Source: three-view drawing plus pictorial views. Frame: mm from the lowest corner of the part. Give positions to 0.01 mm unless a question says otherwise; leave off trailing zeros. Order: outer loops, then holes, each group sorted by start corner. A loop starts at its lowest first (then second) coordinate and runs counter-clockwise, first axis right, second up. Notation, with made-up numbers: M 78.25,64 L 127.25,64 A9 ccw 127.25,76 Z; hole C 61,31.25 d2. An arc over 180 degrees is marked long. Use CSV: the item, a comma, the result in double quotes.
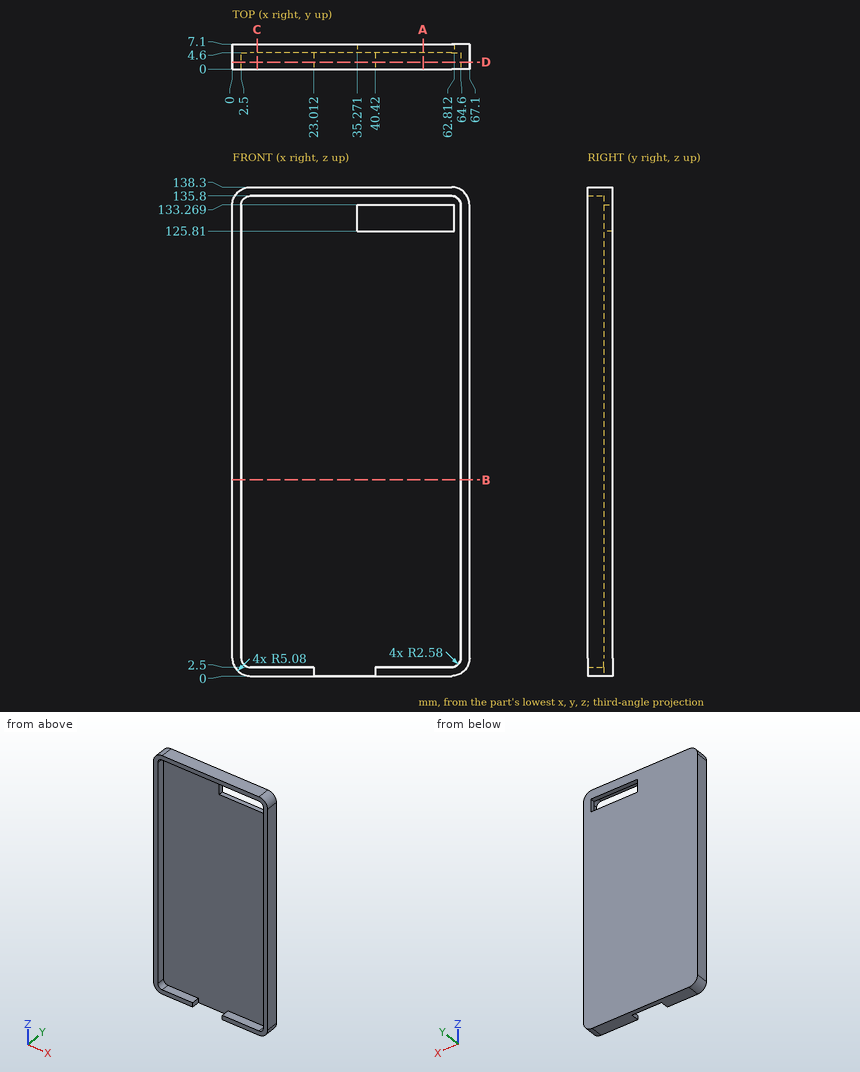
1. Section C-C, the plane x = 7. Return the cut outline in (y, z).
Answer:
outline,"M 0,0 L 7.1,0 L 7.1,138.3 L 0,138.3 L 0,135.8 L 4.6,135.8 L 4.6,2.5 L 0,2.5 Z"
2. Line query: line 1 (Z direction, x = 54.5, y = 6); line 2 (X direction, y = 4, z = 72); line 3 (Z direction, x = 57, y = 0.5). Output: solid intervals per line, ascending.
Answer:
line 1,"0 to 125.81, 133.27 to 138.3"
line 2,"0 to 2.5, 64.6 to 67.1"
line 3,"0 to 2.5, 135.8 to 138.3"
3. Pin query (flat end, axial travel): pin 1 Ø3 at (y, z) = (5.5, 129.5) entering from -X; pin 2 Ø18.5 at (x, z) = (32.5, 92.5) entering from -Y; pin 3 Ø1.2 at (y, z) = (2, 1) entering from -X; pin 4 Ø0.8 at (y, z) = (1.5, 1) entering from +X. Return the tip coordinate at first contact, or that it passes through.
Answer:
pin 1,"x = 0"
pin 2,"y = 4.6"
pin 3,"x = 1.38"
pin 4,"x = 65.52"
4. Section B-B, the plane z = 55.5. Return the cut outline in (x, y).
Answer:
outline,"M 0,0 L 2.5,0 L 2.5,4.6 L 64.6,4.6 L 64.6,0 L 67.1,0 L 67.1,7.1 L 0,7.1 Z"
5. Section A-A, the plane x = 54. Return the cut outline in (y, z).
Answer:
outline,"M 0,0 L 7.1,0 L 7.1,125.81 L 4.6,125.81 L 4.6,2.5 L 0,2.5 Z; M 0,135.8 L 4.6,135.8 L 4.6,133.27 L 7.1,133.27 L 7.1,138.3 L 0,138.3 Z"
6. Section D-D, the plane y = 2. Return the cut outline in (x, z).
Answer:
outline,"M 0,5.08 A5.08 ccw 5.08,0 L 23.01,0 L 23.01,2.5 L 5.08,2.5 A2.58 cw 2.5,5.08 L 2.5,133.22 A2.58 cw 5.08,135.8 L 62.02,135.8 A2.58 cw 64.6,133.22 L 64.6,5.08 A2.58 cw 62.02,2.5 L 40.42,2.5 L 40.42,0 L 62.02,0 A5.08 ccw 67.1,5.08 L 67.1,133.22 A5.08 ccw 62.02,138.3 L 5.08,138.3 A5.08 ccw 0,133.22 Z"
